The listing builds one solid part. Answer for the finished solid, in the listing's coordinates (mm). Face numbers are marked on the shaded views. A direction names the side the tool comes from. Round coordinates to 2 decimals unless told otherwise and drop trailing zeros. Write each loop counter-clockwise with the first axis right and the second up, starting at its lowest first coordinate (ties: lowest second). Pieces come first, ordered by that corner, then holes. Notation, with made-up numbers: (2.5, 31.5) - (10.5, 31.5) arc R20 ccw to (10.5, 49.5) - close; hole circle Ø4 at (79, -13). An arc over 180 degrees is marked (long way). Return JSON: item names as keys, results as strings. Group by question number.
from build123d import *

# Parameters (mm, degrees)
F1_DEPTH = 63.5
F2_DEPTH = 25.4
F3_DEPTH = 7.9375


with BuildPart() as f1:
    # F0 (on Front) → F1 (new body, symmetric)
    with BuildSketch(Plane.XZ):
        Polygon((-12.4777524548, 9.525), (-75.9777524548, 9.525), (-75.9777524548, -9.525), (6.5722475452, -9.525), (6.5722475452, 9.525), (-5.7358437016, 9.525), (-9.173008174, 9.525), align=None)
    extrude(amount=F1_DEPTH, both=True)

    # F0 (on Front) → F2 (join, symmetric)
    with BuildSketch(Plane.XZ):
        with BuildLine():
            Line((-12.4777524548, 26.7462), (-12.4777524548, 9.525))
            Line((-12.4777524548, 9.525), (-9.173008174, 9.525))
            Line((-9.173008174, 9.525), (-5.7358437016, 9.525))
            Line((-5.7358437016, 9.525), (6.5722475452, 9.525))
            Line((6.5722475452, 9.525), (6.5722475452, 26.7462))
            ThreePointArc((6.5722475452, 26.7462), (11.2219273939, 37.9715201513), (22.4472475452, 42.6212))
            Line((22.4472475452, 42.6212), (22.7120646, 42.6212))
            Line((22.7120646, 42.6212), (22.7120646, 61.4994115756))
            Line((22.7120646, 61.4994115756), (18.9874917473, 61.4994115756))
            ThreePointArc((18.9874917473, 61.4994115756), (-3.4427852497, 50.1868021015), (-12.4777524548, 26.7462))
        make_face()
        Polygon((48.1120646, 61.4994115756), (22.7120646, 61.4994115756), (22.7120646, 42.6212), (48.1120646, 42.6212), (48.1120646, 52.3875), align=None)
    extrude(amount=F2_DEPTH, both=True)

    # F0 (on Front) → F3 (join, symmetric)
    with BuildSketch(Plane.XZ):
        with BuildLine():
            add(Edge.make_bspline(
                [(-75.9777524548, 9.525), (-61.7776212541, 25.4792540105), (-62.3238106257, 34.5479376307), (-33.1677066113, 65.9094634104), (2.56170726, 64.6208110814), (18.9874917473, 61.4994115756)],
                knots=[0, 0, 0, 0, 0.3071399643, 0.6175559309, 1, 1, 1, 1], degree=3))
            Line((-75.9777524548, 9.525), (-12.4777524548, 9.525))
            Line((-12.4777524548, 9.525), (-12.4777524548, 26.7462))
            ThreePointArc((-12.4777524548, 26.7462), (-3.4427852497, 50.1868021015), (18.9874917473, 61.4994115756))
        make_face()
    extrude(amount=F3_DEPTH, both=True)

    # F0 (on Front) → F4 (revolve)
    with BuildSketch(Plane.XZ):
        Polygon((48.1120646, 66.675), (48.1120646, 61.4994115756), (48.1120646, 52.3875), (48.1120646, 42.6212), (48.1120646, 38.1), (73.5120646, 38.1), (73.5120646, 66.675), align=None)
    revolve(axis=Axis((48.1120646, 0, 59.53125), (0, 0, 1)))


solid = f1.part
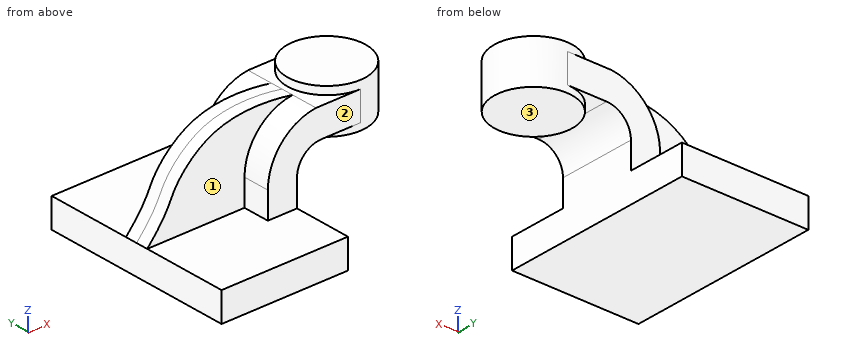
(1) Consider line 1 (Y direction, x = -18, z = 40.5); line 2 (Y direction, x = -4, z = 45); line 3 (X direction, y = -43.5, z = 1.5). Determine where each line is inside the solid, lowest interval first.
(2) Flat-ended cylindrical pins translate along their axes: pin 1 (12 mm diameter, centred on x = -44.5, z = 49, fed in from +Y); pin 2 (20.5 mm diameter, centred on x = 38.5, y = 11.5, fed in from -Z); pin 3 (8 mm diameter, centred on x = -55.5, z = 32.5, fed in from -Y); pin 4 (6 mm diameter, centred on x = -23.5, z = 11.5, fed in from +Y). Find the tip coordinate at first contact, or state that the pin passes through.
(3) Find section B-B (y = 27.5). Write down the section's boundary in (x, z) (3 decimals).
(4) For the marked faces 1, 2 and 3, determine the directions among +Z, -Z, +X, -X, +Y, -Y from which every point of the face is accessible in a straight line to the end or side of a thin tool.
Check sheet entries:
{
 "1": {"line 1": "y = -7.94 to 7.94", "line 2": "y = -25.4 to 25.4", "line 3": "x = -75.98 to 6.57"},
 "2": {"pin 1": "stops at y = 7.94", "pin 2": "stops at z = 38.1", "pin 3": "stops at y = -7.94", "pin 4": "stops at y = 63.5"},
 "3": {"outline": "(-75.978, -9.525) - (6.572, -9.525) - (6.572, 9.525) - (-75.978, 9.525) - close"},
 "4": {"face 1": "+Z, -X, -Y", "face 2": "+Z, +X, -X, -Y", "face 3": "-Z, +X, +Y, -Y"}
}
